Design review of the part built by this model. Coordinates are the model's own, in mm. Round coordinates to 2 decimals unless told otherwise and drop trailing zeros. Write each loop counter-clockwise with the first axis right and the second up, starting at its lowest first coordinate (ties: lowest second). Pieces come first, ordered by that corner, then holes. Notation, with made-up numbers: M 20,23 L 44,23 A16 cw 44,45 Z; hole C -23.75,1.5 d5. An arc over 180 degrees is marked long. One line per question, with ' | ' between items. Start each with the question number.
Item 1: Add section A-A, the plane z = 12. State the section outline as (x, y) points.
Item 2: Add section C-C, the plane z = 0. State the section outline as (x, y) points.
Item 3: For L1, parallel to Y at x = -5, z = 5; L2, parallel to X at y = -10.5, z = 2; L3, parallel to Z at x = 0, y = -8, list the stretches that pass through material, from the lowest coordinate up.
Item 4: Insertion check: pin 1 Ø12 at (y, z) = (-29.5, 13) entering from +X; pin 2 Ø1.5 at (x, z) = (-6.5, 13.5) entering from -Y; pin 3 Ø6 at (y, z) = (-17, 0.5) entering from -X. Each pin has a flat end and moves straight along its axis. Give the tip position at first contact, or say it passes through.
Item 5: Add section B-B, the plane x = 0. State the section outline as (y, z) points.
Item 6: Draft analysis for pull direction Y (two halves, no side actions). For faces 1 (the face through (0, -35, 14)), 2 (the face through (-14.986, -0.493, 0.646)), 3 (the face through (0, -43, 0)), state which applies: released by +Y, released by -Y, zero draft, split by the parting line, or undercut.
Item 7: Add section D-D, the plane y = -38. State the section outline as (x, z) points, and give its area (3 significant figures).
```python
from build123d import *

# Parameters (mm, degrees)
F0_R     = 15
F1_DEPTH = 1
F2_R     = 7
F3_DEPTH = 42
F4_R     = 3
F5_DEPTH = 21
F6_W     = 2
F6_H     = 2
F7_DEPTH = 1.001


with BuildPart() as f1:
    # F0 (on Front) → F1 (new body)
    with BuildSketch(Plane.XZ):
        Circle(F0_R)
    extrude(amount=F1_DEPTH)

    # F2 (on face) → F3 (join)
    with BuildSketch(Plane.XZ.offset(1)):
        Circle(F2_R)
    extrude(amount=F3_DEPTH)

    # F4 (on Top) → F5 (join)
    with BuildSketch(Plane.XY):
        with Locations((0, -38)):
            Circle(F4_R)
    extrude(amount=F5_DEPTH)

    # F6 (on face) → F7 (cut, through all)
    with BuildSketch(Plane.XZ.offset(1)):
        with Locations((15.96663, 0)):
            Rectangle(F6_W, F6_H)
    extrude(amount=-F7_DEPTH, mode=Mode.SUBTRACT)


solid = f1.part
```
Computed values:
1) outline: M -9,-1 L 9,-1 L 9,0 L -9,0 Z; C 0,-38 d6
2) outline: M -15,-1 L -7,-1 L -7,-43 L 7,-43 L 7,-1 L 14.97,-1 L 14.97,0 L -15,0 Z
3) L1: y = -1 to 0 | L2: x = -6.71 to 6.71 | L3: z = -7 to 7
4) pin 1: stops at x = 1.66 | pin 2: stops at y = -1 | pin 3: stops at x = -7
5) outline: M -43,-7 L -1,-7 L -1,-15 L 0,-15 L 0,15 L -1,15 L -1,7 L -35,7 L -35,21 L -41,21 L -41,7 L -43,7 Z
6) face 1: undercut | face 2: zero draft | face 3: released by -Y
7) outline: M -3,6.32 A7 ccw long 3,6.32 L 3,21 L -3,21 Z | area: 239 mm^2
